Can you work these out from the drawing? Everything is in mm from the part's minimum corner. Round coordinates to 2 decimals unless told otherwise and drop trailing zeros. Order: outer loops, then holes, each group sorted by start corner. A loop starts at its lowest first (then second) coordinate and runs counter-clockwise, first axis right, second up. Notation, with made-up numbers: M 52,-18.75 L 104,-18.75 A22 cw 104,-7.75 Z; hole C -18.75,-12 d4. An arc over 180 degrees is marked long. Use one line per item in the form item = value. Start each with the question number.
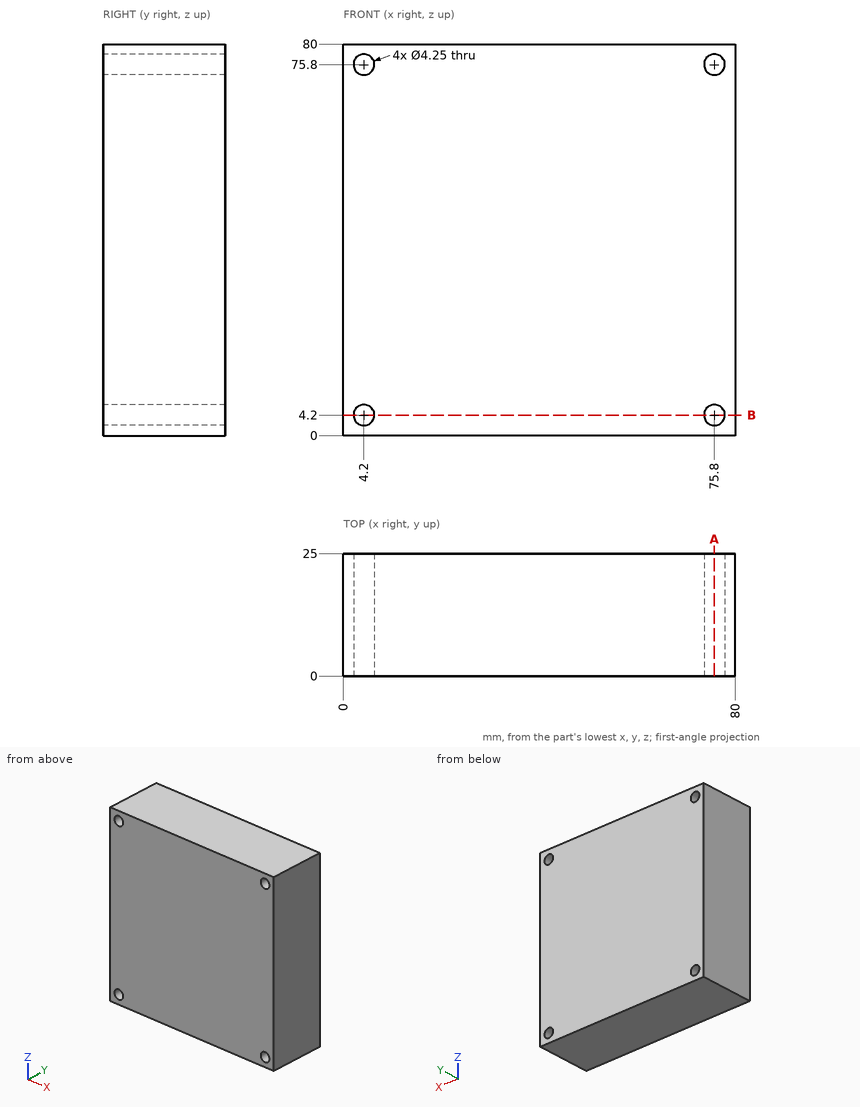
1) If I drill on line 1 (X direction, y = 6.75, z = 75.8) (3 decimals); line 2 (Z direction, x = 77.5, y = 11) (3 decimals), over which ranges is the centre line in solid material (lowest first)?
2) If we section it at B-B on z = 4.2: Write out the boundary of the cut face in (x, y) (3 decimals).
3) If we section it at A-A on x = 75.8: Write out the boundary of the cut face in (y, z) (3 decimals).
Completed:
q1.line_1 = 0 to 2.075, 6.325 to 73.675, 77.925 to 80
q1.line_2 = 0 to 2.925, 5.475 to 74.525, 77.075 to 80
q2.outline = M 0,0 L 2.075,0 L 2.075,25 L 0,25 Z; M 6.325,0 L 73.675,0 L 73.675,25 L 6.325,25 Z; M 77.925,0 L 80,0 L 80,25 L 77.925,25 Z
q3.outline = M 0,0 L 25,0 L 25,2.075 L 0,2.075 Z; M 0,6.325 L 25,6.325 L 25,73.675 L 0,73.675 Z; M 0,77.925 L 25,77.925 L 25,80 L 0,80 Z
